Autodesk Inventor part; units mm, degrees
ref_plane "Work Plane1" through (300.7927, 694.1728, 0) normal (0, 0, 1) x (1, -0.0015, 0)
ref_plane "YZ Plane" through (0, 0, 0) normal (1, 0, 0) x (0, 1, 0)
ref_plane "XZ Plane" through (0, 0, 0) normal (0, 1, 0) x (-1, 0, 0)
ref_plane "Work Plane1" through (300.7927, 694.1728, 0) normal (0, 0, 1) x (1, -0.0015, 0)
sketch "Sketch1" plane through (300.7927, 694.1728, 0) normal (0, 0, 1) x (1, -0.0015, 0)
  line L0 (11.0652, -476.8683) -> (-44.7258, -476.9512) construction
  arc A0 (11.0652, -476.8683) -> (35.1594, -452.7025) centre (11.0294, -452.7384) ccw construction
  line L1 (35.0759, -396.5178) -> (35.1594, -452.7025) construction
  line L2 (32.2566, -396.522) -> (35.0759, -396.5178) construction
  line L3 (32.109, -297.1065) -> (32.2566, -396.522) construction
  line L4 (34.9284, -297.1023) -> (32.109, -297.1065) construction
  line L5 (34.845, -240.9176) -> (34.9284, -297.1023) construction
  arc A1 (34.845, -240.9176) -> (10.6792, -216.8234) centre (10.715, -240.9534) ccw construction
  line L6 (-45.1119, -216.9062) -> (10.6792, -216.8234) construction
  line L7 (-45.1077, -219.7256) -> (-45.1119, -216.9062) construction
  line L8 (-129.6388, -219.8511) -> (-45.1077, -219.7256) construction
  line L9 (-129.643, -217.0317) -> (-129.6388, -219.8511) construction
  line L10 (-166.4983, -217.0864) -> (-129.643, -217.0317) construction
  line L11 (-166.4942, -219.9058) -> (-166.4983, -217.0864) construction
  line L12 (-251.0253, -220.0313) -> (-166.4942, -219.9058) construction
  line L13 (-251.0295, -217.2119) -> (-251.0253, -220.0313) construction
  line L14 (-306.8205, -217.2948) -> (-251.0295, -217.2119) construction
  arc A2 (-306.8205, -217.2948) -> (-330.9146, -241.4606) centre (-306.7847, -241.4247) ccw construction
  line L15 (-330.8312, -297.6453) -> (-330.9146, -241.4606) construction
  line L16 (-328.0118, -297.6411) -> (-330.8312, -297.6453) construction
  line L17 (-327.8643, -397.0566) -> (-328.0118, -297.6411) construction
  line L18 (-330.6836, -397.0608) -> (-327.8643, -397.0566) construction
  line L19 (-330.6002, -453.2455) -> (-330.6836, -397.0608) construction
  arc A3 (-330.6002, -453.2455) -> (-306.4344, -477.3397) centre (-306.4703, -453.2097) ccw construction
  line L20 (-250.6434, -477.2569) -> (-306.4344, -477.3397) construction
  line L21 (-250.6476, -474.4375) -> (-250.6434, -477.2569) construction
  line L22 (-44.73, -474.1318) -> (-250.6476, -474.4375) construction
  line L23 (-44.7258, -476.9512) -> (-44.73, -474.1318) construction
  circle A4 centre (4.6999, -466.5639) radius 1.0795 construction
  circle A5 centre (-300.0998, -467.0164) radius 1.0795 construction
  circle A6 centre (-300.4552, -227.5992) radius 1.0795 construction
  circle A7 centre (4.3445, -227.1467) radius 1.0795 construction
  line L24 (-251.9195, -473.1693) -> (-251.9153, -475.9887)
  line L25 (-251.9153, -475.9887) -> (-306.4363, -476.0697)
  arc A8 (-329.3302, -453.2436) -> (-306.4363, -476.0697) centre (-306.4703, -453.2097) ccw
  line L26 (-329.3302, -453.2436) -> (-329.4118, -398.3289)
  line L27 (-329.4118, -398.3289) -> (-326.5924, -398.3247)
  line L28 (-326.5924, -398.3247) -> (-326.7437, -296.3692)
  line L29 (-326.7437, -296.3692) -> (-329.5631, -296.3734)
  line L30 (-329.5631, -296.3734) -> (-329.6446, -241.4587)
  arc A9 (-306.8186, -218.5648) -> (-329.6446, -241.4587) centre (-306.7847, -241.4247) ccw
  line L31 (-306.8186, -218.5648) -> (-252.2976, -218.4838)
  line L32 (-252.2976, -218.4838) -> (-252.2934, -221.3032)
  line L33 (-252.2934, -221.3032) -> (-165.2223, -221.174)
  line L34 (-165.2223, -221.174) -> (-165.2265, -218.3546)
  line L35 (-165.2265, -218.3546) -> (-130.9111, -218.3036)
  line L36 (-130.9111, -218.3036) -> (-130.9069, -221.123)
  line L37 (-130.9069, -221.123) -> (-43.8358, -220.9938)
  line L38 (-43.8358, -220.9938) -> (-43.84, -218.1744)
  line L39 (-43.84, -218.1744) -> (10.681, -218.0934)
  arc A10 (33.575, -240.9195) -> (10.681, -218.0934) centre (10.715, -240.9534) ccw
  line L40 (33.575, -240.9195) -> (33.6565, -295.8342)
  line L41 (33.6565, -295.8342) -> (30.8371, -295.8384)
  line L42 (30.8371, -295.8384) -> (30.9884, -397.7939)
  line L43 (30.9884, -397.7939) -> (33.8078, -397.7897)
  line L44 (33.8078, -397.7897) -> (33.8894, -452.7044)
  arc A11 (11.0633, -475.5983) -> (33.8894, -452.7044) centre (11.0294, -452.7384) ccw
  line L45 (11.0633, -475.5983) -> (-43.4577, -475.6793)
  line L46 (-43.4577, -475.6793) -> (-43.4619, -472.8599)
  line L47 (-43.4619, -472.8599) -> (-251.9195, -473.1693)
  dimension "d32" = 1.27
extrude "Plate1" add sketch "Sketch1" along normal blind 3.048
sketch "Sketch3" plane through (300.7927, 694.1728, 0) normal (0, 0, -1) x (-1, 0.0015, 0)
  circle A0 centre (300.2757, -466.9836) radius 1.0795 construction
  circle A1 centre (-4.5243, -466.9836) radius 1.0795 construction
  circle A2 centre (-4.5243, -227.5661) radius 1.0795 construction
  circle A3 centre (300.2757, -227.5661) radius 1.0795 construction
  line L0 (-4.5243, -227.5661) -> (300.2757, -227.5661) construction
  line L1 (300.2757, -227.5661) -> (300.2757, -466.9836) construction
  line L2 (300.2757, -466.9836) -> (-4.5243, -466.9836) construction
  line L3 (-4.5243, -466.9836) -> (-4.5243, -227.5661) construction
  line L4 (326.5924, -398.3247) -> (326.7437, -296.3692) construction
  line L5 (326.668, -347.347) -> (300.2757, -347.2749) construction
  line L6 (43.4619, -472.8599) -> (251.9195, -473.1693) construction
  line L7 (165.2265, -218.3546) -> (130.9111, -218.3036) construction
  line L8 (-4.5243, -347.2749) -> (-30.9128, -346.8161) construction
  line L9 (-30.8371, -295.8384) -> (-30.9884, -397.7939) construction
  point P0 (152.4, -347.3112)
  dimension "d2" = 304.8
  dimension "d3" = 239.4175
hole "Mounting_Holes" at (0.1795, 467.0527, 0) at (-0.1759, 227.6355, 0) at (304.6238, 227.183, 0) at (304.9792, 466.6002, 0) direction (0, 0, 1) diameter 3.2766 end through all
sketch "Sketch4" plane through (300.7927, 694.1728, 0) normal (0, 0, -1) x (-1, 0.0015, 0)
  circle A0 centre (4.2521, -424.821) radius 10.541 construction
  line L0 (-33.575, -240.9195) -> (-33.6565, -295.8342)
  line L1 (43.84, -218.1744) -> (-10.681, -218.0934)
  line L2 (-11.0633, -475.5983) -> (43.4577, -475.6793)
  dimension "d11" = 21.082
  dimension "d33" = 38.1
  dimension "d86" = 50.8
hole "Power_Connector" at (295.91, 269.3586, 0) direction (0, 0, 1) diameter 17.4752 end through all
sketch "Sketch7" plane through (300.7927, 694.1728, 3.048) normal (0, 0, 1) x (1, -0.0015, 0)
  line L0 (0.8093, -320.4599) -> (-98.1907, -320.4599)
  line L1 (-98.1907, -320.4599) -> (-98.1907, -278.9599)
  line L2 (-98.1907, -278.9599) -> (0.8093, -278.9599)
  line L3 (0.8093, -278.9599) -> (0.8093, -320.4599)
  line L4 (-165.2265, -218.3546) -> (-130.9111, -218.3036) construction
  line L5 (-43.4619, -472.8599) -> (-251.9195, -473.1693) construction
  line L6 (-43.4619, -472.8599) -> (-251.9195, -473.1693) construction
  line L7 (-147.6907, -473.0146) -> (-147.7272, -448.3951) construction
  point P0 (-299.7619, -694.6186)
  dimension "d40" = 99
  dimension "d41" = 41.5
  dimension "d80" = 152.4
  dimension "d81" = 49.5
extrude "LCD_Cutout" cut sketch "Sketch7" against normal through all
sketch "Sketch8" plane through (300.7927, 694.1728, 3.048) normal (0, 0, 1) x (1, -0.0015, 0)
  line L0 (-1.6907, -327.2099) -> (-95.6907, -327.2099) construction
  line L1 (-95.6907, -327.2099) -> (-95.6907, -272.2099) construction
  line L2 (-95.6907, -272.2099) -> (-1.6907, -272.2099) construction
  line L3 (-1.6907, -272.2099) -> (-1.6907, -327.2099) construction
  line L4 (-48.6907, -327.2099) -> (-48.6907, -320.4599) construction
  line L5 (0.8093, -320.4599) -> (-98.1907, -320.4599) construction
  line L6 (-98.1907, -278.9599) -> (0.8093, -278.9599) construction
  line L7 (-48.6907, -278.9599) -> (-48.6907, -272.2099) construction
  point P0 (-299.7619, -694.6186)
  dimension "d45" = 94
  dimension "d46" = 55
hole "LCD_Holes" at (298.6163, 366.9658, 3.048) at (204.6164, 367.1053, 3.048) at (204.698, 422.1053, 3.048) at (298.6979, 421.9657, 3.048) direction (0, 0, -1) diameter 3.2766 end through all
sketch "Sketch9" plane through (300.7927, 694.1728, 3.048) normal (0, 0, 1) x (1, -0.0015, 0)
  circle A0 centre (-4.2521, -424.821) radius 9.0607
  line L0 (30.8371, -295.8384) -> (30.9884, -397.7939)
  point P0 (-299.7619, -694.6186)
  point P1 (-55.0521, -386.721)
  dimension "d84" = 50.8
  dimension "d85" = 38.1
hole "Pickle_Switch" at (245.1666, 307.5339, 3.048) direction (0, 0, -1) diameter 12 end through all
sketch "Sketch10" plane through (300.7927, 694.1728, 3.048) normal (0, 0, 1) x (1, -0.0015, 0)
  line L0 (-15.1907, -253.5599) -> (-82.1907, -253.5599) construction
  line L1 (-98.1907, -278.9599) -> (0.8093, -278.9599) construction
  line L2 (-48.6907, -278.9599) -> (-48.6907, -253.5599) construction
  line L3 (0.8093, -278.9599) -> (0.8093, -320.4599) construction
  point P0 (-299.7619, -694.6186)
  dimension "d62" = 16
  dimension "d63" = 25.4
hole "Pushbuttons" at (285.2256, 440.6357, 3.048) at (251.7257, 440.6855, 3.048) at (218.2257, 440.7352, 3.048) direction (0, 0, -1) diameter 17.5006 end through all
sketch "Sketch11" plane through (300.7927, 694.1728, 3.048) normal (0, 0, 1) x (1, -0.0015, 0)
  circle A0 centre (-4.2521, -424.821) radius 9.0607 construction
  circle A1 centre (-55.0521, -386.721) radius 6 construction
  line L0 (-4.2521, -424.821) -> (-4.2521, -386.721) construction
  point P0 (-299.7619, -694.6186)
  dimension "d71" = 38.1
hole "Air_Coupler" at (295.9666, 307.4585, 3.048) direction (0, 0, -1) diameter 8.89 depth 3.048 tip angle 118
sketch "Sketch12" plane through (300.7927, 694.1728, 3.048) normal (0, 0, 1) x (1, -0.0015, 0)
  line L0 (-250.9997, -426.9053) -> (-287.5757, -426.9053)
  line L1 (-287.5757, -426.9053) -> (-287.5757, -405.3661)
  line L2 (-287.5757, -405.3661) -> (-250.9997, -405.3661)
  line L3 (-250.9997, -405.3661) -> (-250.9997, -426.9053)
  circle A0 centre (-300.2757, -227.5661) radius 1.6383 construction
  point P0 (-299.7619, -694.6186)
  dimension "d87" = 36.576
  dimension "d88" = 21.5392
  dimension "d89" = 177.8
  dimension "d90" = 12.7
extrude "Powerpole_Cutout" cut sketch "Sketch12" against normal blind 3.048
sketch "Sketch13" plane through (300.7927, 694.1728, 3.048) normal (0, 0, 1) x (1, -0.0015, 0)
  line L0 (-15.3261, -339.5099) -> (-44.6761, -339.5099) construction
  line L1 (30.8371, -295.8384) -> (30.9884, -397.7939) construction
  line L2 (0.8093, -320.4599) -> (-98.1907, -320.4599) construction
  point P0 (-299.7619, -694.6186)
  dimension "d93" = 46.228
  dimension "d94" = 29.35
  dimension "d95" = 19.05
hole "Fan Bracket" at (284.9626, 354.686, 3.048) at (255.6126, 354.7296, 3.048) direction (0, 0, -1) diameter 3.2766 end through all
equation "\"d9\" = Thickness"
equation "\"d43\" = Thickness"
equation "\"d45\" = LCD_PCB_Horizontal_Hole_Spacing"
equation "\"d46\" = LCD_PCB_Vertical_Hole_Spacing"
equation "\"d47\" = LCD_Cover_Hole_Diameter"
equation "\"d60\" = Thickness"
equation "\"d69\" = Thickness"
equation "\"d77\" = Thickness"
equation "\"d91\" = Thickness"
equation "\"d94\" = Bracket_Hole_Spacing"
equation "\"d101\" = Thickness"
equation "\"d81\" = 0.5 * d40"
equation "\"BendRadius\" = Thickness"
equation "\"BendReliefWidth\" = Thickness"
equation "\"BendReliefDepth\" = 0.5 * Thickness"
equation "\"CornerReliefSize\" = 4 * Thickness"
equation "\"MinimumRemnant\" = 2 * Thickness"
equation "\"TransitionRadius\" = BendRadius"
equation "\"JacobiRadiusSize\" = BendRadius"
equation "\"GapSize\" = Thickness"
equation "\"d1\" = BendRadius"
properties part number "Panel" material "Acetal Resin, Black"
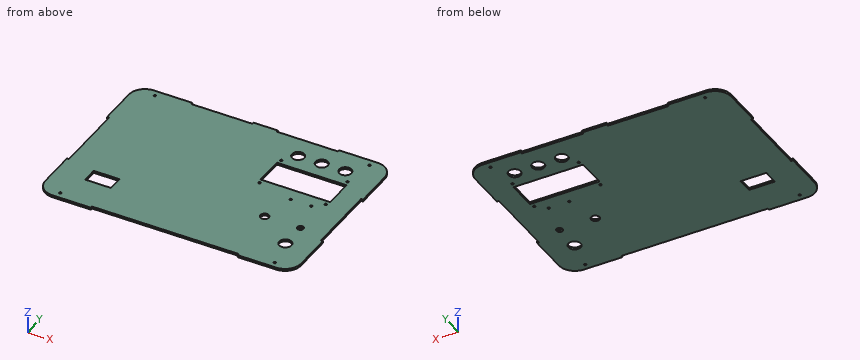
Geometry check sheet. Reference: the model listing, model coordinates, mm. Give positions to 0.01 mm unless a question says otherwise; leave off trailing zeros. Loops run counter-clockwise (first coordinate to the right, second up) from the corner with the lowest first, then second, coordinate; pieces in that order, holes last. Notation, with made-up numbers: (64.5, 79.25) - (111.5, 79.25) arc R21 cw to (111.5, 110.25) - close; hole circle Ø3 at (-8, 62.5). An arc over 180 degrees is marked (long way). Use CSV: the item, a comma, the result in double quotes. Start each with the question number.
Q1. Section check A-A, the plane x = 44.5. Record the cut outline in (y, z).
Q2. Scan lines: probe 1 along Y at (x, z) = (29.5, 1); probe 2 along X at (y, z) = (388.5, 1); probe 3 along Y at (x, z) = (268.5, 2.05). Record each from-to range of solid material in increasing order. Write a range as from..to.
Q3. Section check C-C, the plane x = 108. Record the cut outline in (y, z).
Q4. Go/stop test with flat-tipped pins: pin 1 Ø0.9 at (x, z) = (79.5, 2) entering from +Y; pin 2 Ø1.5 at (y, z) = (430.5, 1) entering from -X; pin 3 Ø0.9 at (y, z) = (346.5, 2) entering from +X. Record where each tip stops, or that it passes through.
Q5. Section check B-B, the plane z = 1.15. Count the separate pieces of the cut face and the enclosed holes in it, and give its area (3 significant figures).
Findings below:
1,outline,"(218.56, 0) - (267.65, 0) - (267.65, 3.05) - (218.56, 3.05) - close; (289.19, 0) - (476.07, 0) - (476.07, 3.05) - (289.19, 3.05) - close"
2,probe 1,"y = 218.56..267.67, 289.21..476.07"
2,probe 2,"x = -26.4..202.14, 301.14..331.19"
2,probe 3,"y = 218.56..373.76, 415.26..476.06"
3,outline,"(221.38, 0) - (473.25, 0) - (473.25, 3.05) - (221.38, 3.05) - close"
4,pin 1,"stops at y = 473.25"
4,pin 2,"stops at x = -29.21"
4,pin 3,"stops at x = 331.19"
5,separate pieces,"1"
5,enclosed holes,"18"
5,area,"85,300 mm^2"
